Input: dimensioned drawing with shaded views. Units: mm. Origin: part minimum x, y, z. A direction names the side the tool comes from. Give positions to 0.01 mm unless a question says otherwise; leave off trailing zeros. Write each loop counter-clockwise with the first axis right and the second up, starting at its lowest first coordinate (ties: lowest second). Pieces come first, ordered by that corner, then holes. Notation, with made-up numbers: (-8, -1.5) -> (34, -1.5) arc R31 ccw to (34, 36.5) -> close; hole circle Ø10 at (9.5, 9.5). An arc over 180 degrees is marked (long way). Answer as a JSON object with one key per item and string values.
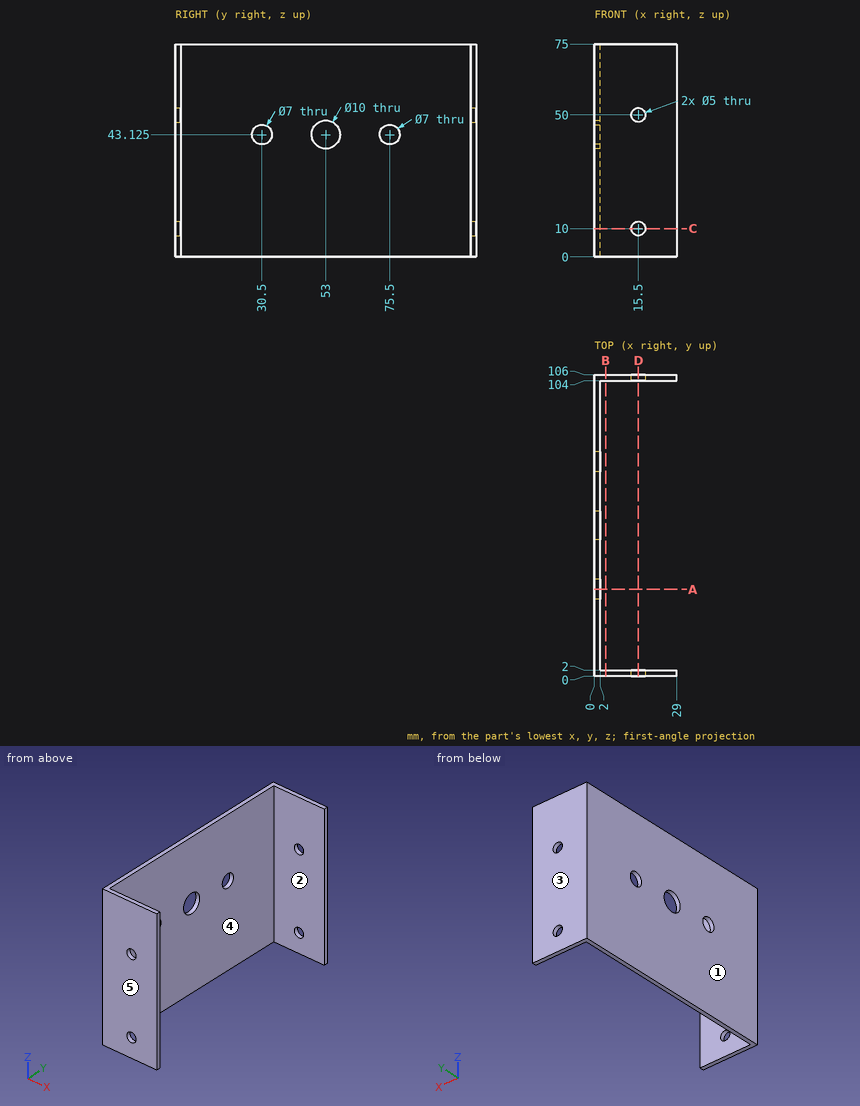
Q1. Material intervals for L1, parallel to Y at x = 19.75, z = 57.5; L2, parallel to Z at x = 15.5, y = 105.3; L3, parallel to X at y = 54, z = 59, sorted ascending. Write a range as from..to.
Values:
{"L1": "0..2, 104..106", "L2": "0..7.5, 12.5..47.5, 52.5..75", "L3": "0..2"}
Q2. Set-up query: the marked faces 4 and 5. Return all of +Z, -Z, +X, -X, +Y, -Y with unobstructed straight access to the full face (end or side cutting, diameter ignored); none if empty.
Values:
{"face 4": "+Z, -Z, +X", "face 5": "+Z, -Z, +X, -X, -Y"}
Q3. First-contact query: P1, Ø3, axis at x = 5, y = 83.5, coming from the +Z side; P2, Ø12, axis at y = 41.5, z = 28.5, coming from the +X side. Flat tips, straight axial feed; report the tip coordinate or a pass-through.
Values:
{"P1": "through", "P2": "x = 2"}
Q4. Cut plane A-A (y = 30.5). Return the cut outline in (x, z) (3 decimals), and give its area (3 significant figures).
Values:
{"outline": "(0, 0) -> (2, 0) -> (2, 39.625) -> (0, 39.625) -> close; (0, 46.625) -> (2, 46.625) -> (2, 75) -> (0, 75) -> close", "area": "136 mm²"}
Q5. Mould query, pull axis Y, two halves, no side actions, for the marked faces 1, 2 and 3. Classes: pulls with the +Y half, pulls with the -Y half, needs draft (parallel to the pull), parting line crosses it, or undercut.
Values:
{"face 1": "needs draft", "face 2": "undercut", "face 3": "pulls with the +Y half"}
Q6. Cut plane C-C (z = 10). Return the cut outline in (x, y).
Values:
{"outline": "(0, 0) -> (13, 0) -> (13, 2) -> (2, 2) -> (2, 104) -> (13, 104) -> (13, 106) -> (0, 106) -> close; (18, 0) -> (29, 0) -> (29, 2) -> (18, 2) -> close; (18, 104) -> (29, 104) -> (29, 106) -> (18, 106) -> close"}
Q7. Cut plane B-B (x = 4). Return the cut outline in (y, z), and give its area (3 significant figures).
Values:
{"outline": "(0, 0) -> (2, 0) -> (2, 75) -> (0, 75) -> close; (104, 0) -> (106, 0) -> (106, 75) -> (104, 75) -> close", "area": "300 mm²"}
Q8. Cut plane D-D (x = 15.5). Return the cut outline in (y, z), and give its area (3 significant figures).
Values:
{"outline": "(0, 0) -> (2, 0) -> (2, 7.5) -> (0, 7.5) -> close; (0, 12.5) -> (2, 12.5) -> (2, 47.5) -> (0, 47.5) -> close; (0, 52.5) -> (2, 52.5) -> (2, 75) -> (0, 75) -> close; (104, 0) -> (106, 0) -> (106, 7.5) -> (104, 7.5) -> close; (104, 12.5) -> (106, 12.5) -> (106, 47.5) -> (104, 47.5) -> close; (104, 52.5) -> (106, 52.5) -> (106, 75) -> (104, 75) -> close", "area": "260 mm²"}
